```python
from build123d import *

# Parameters (mm, degrees)
F0_R          = 2.5
F1_DEPTH      = 2.5
F2_W          = 10.5
F2_H          = 30
F3_DEPTH      = 5.001
F5_DEPTH      = 30.5475219467
F5_DEPTH_BACK = 25.001
F6_R          = 9.99999
F7_R          = 2


# Not quite as in the source:
# - a fillet or chamfer is up to 0.001 mm smaller than in the source, because OpenCascade refuses the exact size


with BuildPart() as f1:
    # F0 (on Top) → F1 (new body, symmetric)
    with BuildSketch(Plane.XY):
        with BuildLine():
            ThreePointArc((-4.6363826998, 28.0052303576), (-7.3366406052, 24.8446324714), (-10.8006642439, 22.5465219467))
            ThreePointArc((-10.8006642439, 22.5465219467), (0, -25), (10.8006642439, 22.5465219467))
            ThreePointArc((10.8006642439, 22.5465219467), (7.3366406052, 24.8446324714), (4.6363826998, 28.0052303576))
            ThreePointArc((4.6363826998, 28.0052303576), (0, 30.5465219467), (-4.6363826998, 28.0052303576))
        make_face()
        with Locations((0, 25.0465219467)):
            Circle(F0_R, mode=Mode.SUBTRACT)
    extrude(amount=F1_DEPTH, both=True)

    # F2 (on face) → F3 (cut, through all)
    with BuildSketch(Plane.XY.offset(2.5)):
        Rectangle(F2_W, F2_H)
    extrude(amount=-F3_DEPTH, mode=Mode.SUBTRACT)

    # F4 (on Front) → F5 (cut, two sides)
    with BuildSketch(Plane.XZ) as f5_sk:
        with BuildLine():
            ThreePointArc((0, 6.579392902), (31.2333147735, 20), (0, 33.420607098))
            ThreePointArc((0, 33.420607098), (-31.2333147735, 20), (0, 6.579392902))
        make_face()
    extrude(amount=-F5_DEPTH, mode=Mode.SUBTRACT)
    extrude(f5_sk.sketch, amount=F5_DEPTH_BACK, mode=Mode.SUBTRACT)

    # F6 (radius 10 in the source; OpenCascade refuses exactly that, so slightly less here)
    f6_edges = [f1.edges().sort_by_distance(p)[0] for p in [
        (-6.733315, 0.666562, 2.5),
        (-18.733315, 0, 2.5),
        (6.733315, 0.666562, 2.5),
        (18.733315, 0, 2.5),
    ]]
    fillet(f6_edges, radius=F6_R)

    # F7
    f7_edges = [f1.edges().sort_by_distance(p)[0] for p in [
        (5.25, 15, 0),
        (5.25, -15, 0),
        (-5.25, -15, 0),
        (-5.25, 15, 0),
    ]]
    fillet(f7_edges, radius=F7_R)


solid = f1.part
```
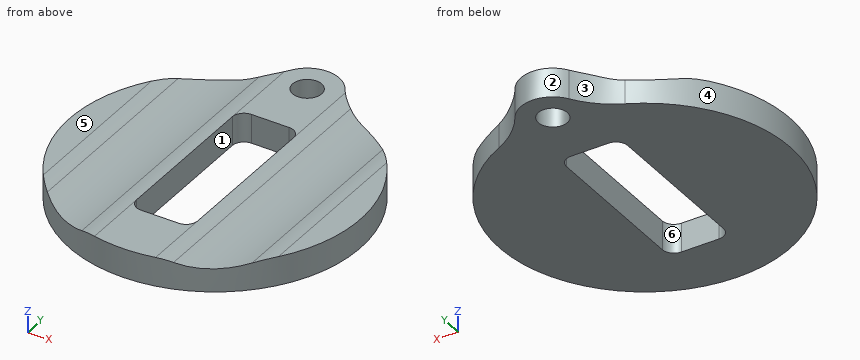
Here's how the part is built. I have some questions about the finished solid (model axes, mm). Face numbers are marked on the shaded views. A direction names the side the tool comes from. Give positions to 0.01 mm unless a question says otherwise; leave off trailing zeros. Write each loop counter-clockwise with the first axis right and the second up, starting at its lowest first coordinate (ties: lowest second). Pieces come first, ordered by that corner, then holes.
(1) Imagine slicing it at B-B, the plane x = 0. Write out the boundary of the cut face in (y, z).
Output values:
outline: (-25, -2.5) - (-15, -2.5) - (-15, 2.5) - (-25, 2.5) - close; (15, -2.5) - (22.55, -2.5) - (22.55, 2.5) - (15, 2.5) - close; (27.55, -2.5) - (30.55, -2.5) - (30.55, 2.5) - (27.55, 2.5) - close
(2) Imagine slicing it at C-C, the plane z = -0.3. Write out the boundary of the cut face in (x, y).
Output values:
outline: (-10.8, 22.55) arc R25 ccw (long way) to (10.8, 22.55) arc R15 cw to (4.64, 28.01) arc R5.5 ccw to (-4.64, 28.01) arc R15 cw to start; hole (-5.25, -13) arc R2 ccw to (-3.25, -15) - (3.25, -15) arc R2 ccw to (5.25, -13) - (5.25, 13) arc R2 ccw to (3.25, 15) - (-3.25, 15) arc R2 ccw to (-5.25, 13) - close; hole circle Ø5 at (0, 25.05)
(3) Thinking about a two-plate mould opening in X: for the marked faces 3, 4, 5 and 6, which applies, pulls with the +X half, pulls with the -X half, needs draft (parallel to the pull), parting line crosses it, or undercut?
Output values:
face 3: pulls with the -X half
face 4: parting line crosses it
face 5: needs draft
face 6: undercut
(4) If I drill on L1, parallel to Y at x = 0, z = 1.2; L2, parallel to Y at x = -1.5, z = -0.95; L3, parallel to Z at x = -5.5, y = 1.5, over which ranges is the centre line in solid material (lowest first)?
Output values:
L1: y = -25 to -15, 15 to 22.55, 27.55 to 30.55
L2: y = -24.95 to -15, 15 to 23.05, 27.05 to 30.34
L3: z = -2.5 to 2.5
(5) Imagine slicing it at D-D, the plane y = 21. Write out the boundary of the cut face in (x, z).
Output values:
outline: (-13.56, -2.5) - (13.56, -2.5) - (13.56, 1.52) arc R18.5 cw to (7.88, 2.15) arc R10 ccw to (5.25, 2.5) - (-5.25, 2.5) arc R10 ccw to (-7.88, 2.15) arc R18.5 cw to (-13.56, 1.52) - close
(6) On a 3-axis mill with a long thin cutter (end or side, diameter ignored), from which of +Z, -Z, +X, -X, +Y, -Y can I reach the whole of each face in a straight line? I mean the marked faces 1 and 2. Say none if no direction works.
Output values:
face 1: +Z, -Z
face 2: +Z, -Z, +Y
(7) Will these pins go through, and if not, where does the flat tip stop? pin 1 (5 mm diameter, centred on x = 13.5, y = 14.5, fed in from +Z); pin 2 (3 mm diameter, centred on x = 0, y = 25.05, fed in from +Z); pin 3 (1 mm diameter, centred on y = -8, z = 1, fed in from -X); pin 4 (3 mm diameter, centred on x = -8, z = 0, fed in from -Y).
Output values:
pin 1: stops at z = 1.79
pin 2: passes through
pin 3: stops at x = -23.85
pin 4: stops at y = -24.14
